Autodesk Fusion 360 part; units mm, degrees
sketch "Sketch1" plane through (0, 0, 0) normal (0, 0, 1) x (1, 0, 0)
  line L0 (-10, 20) -> (10, 20)
  circle A0 centre (-4.5, 24.24) radius 1.5
  line L1 (0, 24.24) -> (0, 20) construction
  circle A1 centre (4.5, 24.24) radius 1.5
  line L2 (4.5, 24.24) -> (-4.5, 24.24) construction
  line L3 (0, 0) -> (10.6295, 0) construction
  line L4 (0, 0) -> (0, 5.1011) construction
  line L5 (10, -20) -> (-10, -20)
  line L6 (10, 20) -> (10, -20)
  line L7 (-10, -20) -> (10, 20) construction
  line L8 (22, -29) -> (22, 29)
  line L9 (-10, -20) -> (-10, 20)
  line L10 (10, -20) -> (-10, 20) construction
  line L11 (-20, -29) -> (-20, 29)
  line L12 (22, 29) -> (-20, 29)
  line L13 (22, -29) -> (-20, -29)
  circle A2 centre (-4.5, -24.24) radius 1.5
  circle A3 centre (4.5, -24.24) radius 1.5
  circle A4 centre (-13, -17) radius 1.25
  circle A5 centre (-13, -17) radius 2.5 construction
  line L14 (-10, -20) -> (-13, -20) construction
  line L15 (-13, -20) -> (-13, -17) construction
  line L16 (-10.5, -17) -> (-10, -17) construction
  line L17 (-15.5, -17) -> (-20, -17) construction
  line L18 (-10.5, -17) -> (-13, -17) construction
  circle A6 centre (14.1, -24.9) radius 1.25
  line L19 (14.1, -24.9) -> (14.1, -11.9) construction
  circle A7 centre (14.1, -11.9) radius 1.25
  circle A8 centre (14.1, -11.9) radius 4.1 construction
  circle A9 centre (14.1, -24.9) radius 4.1 construction
  dimension "d3" = 20
  dimension "d4" = 40
  dimension "d6" = 9
  dimension "d8" = 4.24
  dimension "d9" = 3
  dimension "d10" = 3
  dimension "d18" = 9
  dimension "d19" = 10
  dimension "d20" = 12
  dimension "d21" = 2.5
  dimension "d22" = 5
  dimension "d23" = 3
  dimension "d26" = 3
  dimension "d29" = 0.5
  dimension "d31" = 4.5
  dimension "d32" = 2.5
  dimension "d33" = 2.5
  dimension "d34" = 13
  dimension "d35" = 8.2
  dimension "d36" = 8.2
extrude "Extrude1" add sketch "Sketch1" along normal blind 3
fillet "Fillet1" radius 0.75 4 edges at (-10, -20, 1.5) (10, -20, 1.5) (10, 20, 1.5) (-10, 20, 1.5)
fillet "Fillet2" radius 1 4 edges at (-20, -29, 1.5) (22, -29, 1.5) (-20, 29, 1.5) (22, 29, 1.5)
sketch "Laser" plane through (0, 0, 3) normal (0, 0, 1) x (-1, 0, 0)
  arc A0 (-22, -28) -> (-21, -29) centre (-21, -28) ccw
  line L0 (-21, -29) -> (19, -29)
  arc A1 (19, -29) -> (20, -28) centre (19, -28) ccw
  line L1 (20, -28) -> (20, 28)
  arc A2 (20, 28) -> (19, 29) centre (19, 28) ccw
  line L2 (19, 29) -> (-21, 29)
  arc A3 (-21, 29) -> (-22, 28) centre (-21, 28) ccw
  line L3 (-22, 28) -> (-22, -28)
  circle A4 centre (-14.1, 11.9) radius 1.25
  circle A5 centre (4.5, -24.24) radius 1.5
  circle A6 centre (4.5, 24.24) radius 1.5
  circle A7 centre (13, 17) radius 1.25
  circle A8 centre (-4.5, 24.24) radius 1.5
  circle A9 centre (-14.1, 24.9) radius 1.25
  line L4 (-9.25, 20) -> (9.25, 20)
  arc A10 (10, 19.25) -> (9.25, 20) centre (9.25, 19.25) ccw
  line L5 (10, 19.25) -> (10, -19.25)
  arc A11 (9.25, -20) -> (10, -19.25) centre (9.25, -19.25) ccw
  line L6 (9.25, -20) -> (-9.25, -20)
  arc A12 (-10, -19.25) -> (-9.25, -20) centre (-9.25, -19.25) ccw
  line L7 (-10, -19.25) -> (-10, 19.25)
  arc A13 (-9.25, 20) -> (-10, 19.25) centre (-9.25, 19.25) ccw
  circle A14 centre (-4.5, -24.24) radius 1.5
  line L8 (-14.1, 11.9) -> (-14.1, 24.9) construction
  line L9 (-16, 22) -> (-12.2, 22)
  line L10 (-12.2, 22) -> (-12.2, 14.8)
  line L11 (-12.2, 14.8) -> (-16, 14.8)
  line L12 (-16, 14.8) -> (-16, 22)
  line L13 (-16, 22) -> (-12.2, 14.8) construction
  line L14 (-12.2, 22) -> (-16, 14.8) construction
  point P0 (-14.1, 18.4)
equation "d20 = 8 mm + 4 mm"
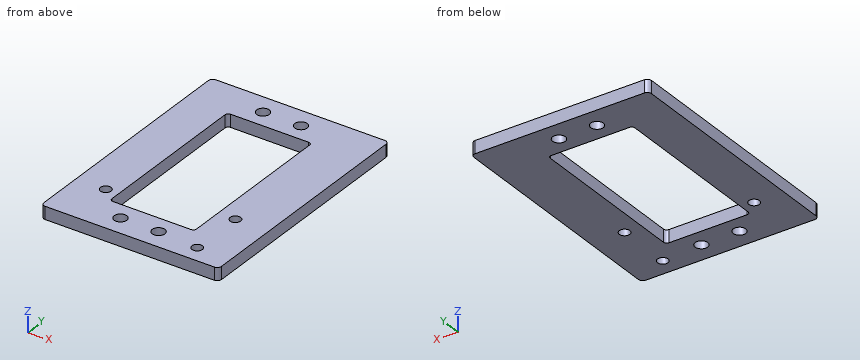
Read the model definition and answer for the solid it produces. Units are mm, in the model's axes. Round coordinates to 2 decimals unless told otherwise and drop trailing zeros. Loops run counter-clockwise (first coordinate to the right, second up) from the corner with the lowest first, then second, coordinate; pieces in that order, holes last. Notation, with made-up numbers: (84.25, 56.25) - (92.25, 56.25) arc R20 cw to (92.25, 73.25) - close; hole circle Ø8 at (15.25, 66). An arc over 180 degrees is marked (long way). One line per question, with ' | ' between items. Start each with the question number.
Q1. Find the intervals of material crossed by L1, parallel to Y at x = 14.1, z = 1.75; L2, parallel to Y at x = 4.5, z = 0.6; L3, parallel to X at y = -2.5, z = 1.95, in increasing order.
Q2. Section B-B on x = -13 is taken. Give the vertices of the cut face in (y, z).
Q3. Section D-D on y = 12 is taken. Give the vertices of the cut face in (x, z), plus the area to 3 significant figures.
Q4. Section A-A on y = 24.24 is taken. Give the vertices of the cut face in (x, z), plus the area to 3 significant figures.
Q5. Section C-C on z = 0.6 is taken. Count the separate pieces of the cut face and the enclosed holes in it, plus the area to 3 significant figures.
Established:
1) L1: -29 to -26.15, -23.65 to -13.15, -10.65 to 29 | L2: -29 to -25.74, -22.74 to -20, 20 to 22.74, 25.74 to 29 | L3: -20 to -10, 10 to 22
2) outline: (-29, 0) - (-18.25, 0) - (-18.25, 3) - (-29, 3) - close; (-15.75, 0) - (29, 0) - (29, 3) - (-15.75, 3) - close
3) outline: (-20, 0) - (-10, 0) - (-10, 3) - (-20, 3) - close; (10, 0) - (22, 0) - (22, 3) - (10, 3) - close | area: 66.0 mm²
4) outline: (-20, 0) - (-6, 0) - (-6, 3) - (-20, 3) - close; (-3, 0) - (3, 0) - (3, 3) - (-3, 3) - close; (6, 0) - (22, 0) - (22, 3) - (6, 3) - close | area: 108 mm²
5) separate pieces: 1 | enclosed holes: 8 | area: 1,590 mm²
